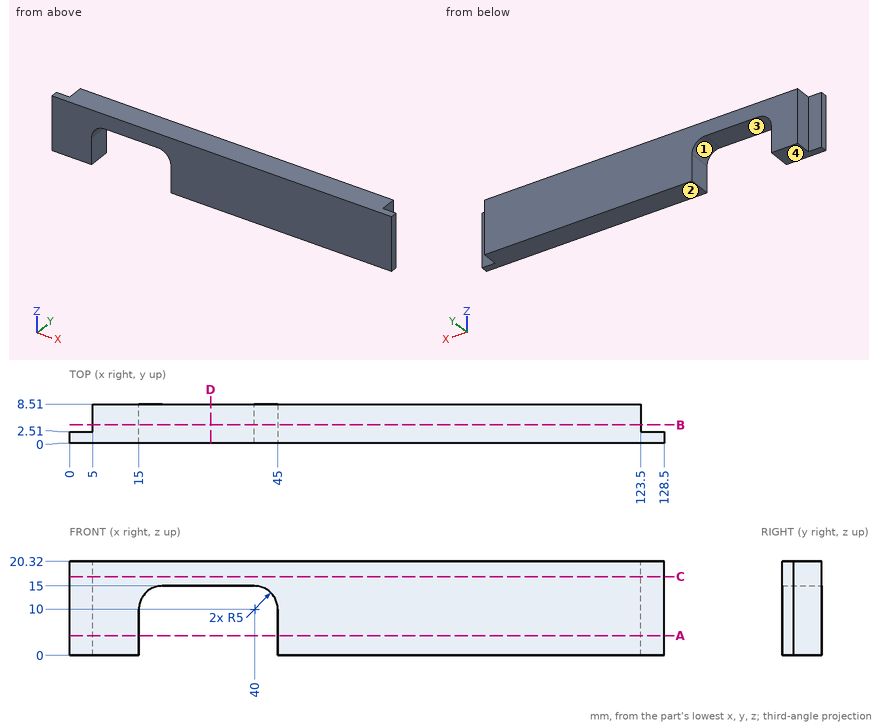
Study the drawing (mm; zero at the part's minimum x, y, z) and answer. A direction names the side the tool comes from. Give positions to 0.01 mm unless a question says otherwise; leave off trailing zeros. Loops run counter-clockwise (first coordinate to the right, second up) from the corner with the lowest first, then second, coordinate; pieces in that order, holes last. Notation, with made-up numbers: (-37.5, 34) - (8.5, 34) arc R13 ccw to (8.5, 46) - close; hole circle Ø7 at (58.25, 24). An arc over 180 degrees is marked (long way). Return JSON: item names as keys, results as strings. Group by question number.
1. Which of the six approach directions +Z, -Z, +X, -X, +Y, -Y give full straight-line access (tool end or side, diameter ignored) to the marked faces 3 and 4?
2. Find section C-C (z = 17). Write down the section's boundary in (x, y), then the cut area to 3 significant figures.
3. Determine the mould class of the marked faces 1 and 2 for opening direction X: pulls with the +X half, pulls with the -X half, needs draft (parallel to the pull), parting line crosses it, or undercut.
4. Given pin 1 Ø2.5 at (x, z) = (127, 10) entering from +Y; pin 2 Ø1.5 at (x, z) = (17.5, 11) entering from +Y; pin 3 Ø1.8 at (y, z) = (5.5, 14.5) entering from -X; pin 4 Ø5 at (y, z) = (6.5, 7.5) entering from +X, each flat-ended and moving along its own axis, determine where each tip first touches the part or whether it passes through.
5. Find section D-D (x = 30.5). Write down the section's boundary in (y, z).
6. Find section B-B (y = 4). Write down the section's boundary in (x, z).
7. Find section A-A (z = 4.25). Write down the section's boundary in (x, y).
8. Straight lines are drawn through the part: line 1 (X direction, y = 3.5, z = 2.5); line 2 (X direction, y = 1, z = 2.5); line 3 (Z direction, x = 27, y = 4). For each, find the intervals that lie inside material, in ascending order. Write a range as [from, to].
Verdict:
{
 "1": {"face 3": "-Z, +Y, -Y", "face 4": "-Z, +X, -X, +Y, -Y"},
 "2": {"outline": "(0, 0) - (128.5, 0) - (128.5, 2.51) - (123.5, 2.51) - (123.5, 8.51) - (5, 8.51) - (5, 2.51) - (0, 2.51) - close", "area": "1,030 mm^2"},
 "3": {"face 1": "undercut", "face 2": "needs draft"},
 "4": {"pin 1": "stops at y = 2.51", "pin 2": "passes through", "pin 3": "stops at x = 5", "pin 4": "stops at x = 123.5"},
 "5": {"outline": "(0, 15) - (8.51, 15) - (8.51, 20.32) - (0, 20.32) - close"},
 "6": {"outline": "(5, 0) - (15, 0) - (15, 10) arc R5 cw to (20, 15) - (39.95, 15) arc R5 cw to (45, 10) - (45, 0) - (123.5, 0) - (123.5, 20.32) - (5, 20.32) - close"},
 "7": {"outline": "(0, 0) - (15, 0) - (15, 8.51) - (5, 8.51) - (5, 2.51) - (0, 2.51) - close; (45, 0) - (128.5, 0) - (128.5, 2.51) - (123.5, 2.51) - (123.5, 8.51) - (45, 8.51) - close"},
 "8": {"line 1": "x = [5, 15], [45, 123.5]", "line 2": "x = [0, 15], [45, 128.5]", "line 3": "z = [15, 20.32]"}
}
